```python
from build123d import *

# Parameters (mm, degrees)
CBORE_FOR_M2_SHCS1_AT_2_COUNT = 2
CBORE_FOR_M2_SHCS1_AT_2_PITCH = 6.363961031
CBORE_FOR_M2_SHCS1_AT_3_COUNT = 2
CBORE_FOR_M2_SHCS1_AT_3_PITCH = 9
CBORE_FOR_M2_SHCS1_AT_4_COUNT = 2
CBORE_FOR_M2_SHCS1_AT_4_PITCH = 6.363961031


with BuildPart() as part:
    # Sketch1 → Revolve1 (revolve)
    with BuildSketch(Plane.XY, mode=Mode.PRIVATE) as revolve1_sk:
        Polygon((0, 0), (8, 0), (8, 3.5), (2, 3.5), (2, 14.5), (0, 14.5), align=None)
    revolve(revolve1_sk.sketch.rotate(Axis((0, 14.5, 0), (0, -1, 0)), 180), axis=Axis((0, 14.5, 0), (0, -1, 0)))

    # Sketch4 → CBORE for M2 SHCS1 (revolve, cut)
    with BuildSketch(Plane(origin=(-4.5, 3.5, 0), x_dir=(0, 0, 1), z_dir=(1, 0, 0))):
        Polygon((0, 0), (0, 3.5), (1.2, 3.5), (1.2, 2), (2.2, 2), (2.2, 0.025), (2.225, 0), align=None)
    cbore_for_m2_shcs1 = revolve(axis=Axis((-4.5, 9.85, 0), (0, -1, 0)), mode=Mode.SUBTRACT)

    # CBORE for M2 SHCS1 at 2: CBORE for M2 SHCS1 ×2
    with Locations(*[Vector(0.7071067811865476, 0, -0.7071067811865476) * (i * CBORE_FOR_M2_SHCS1_AT_2_PITCH) for i in range(1, CBORE_FOR_M2_SHCS1_AT_2_COUNT)]):
        add(cbore_for_m2_shcs1, mode=Mode.SUBTRACT)

    # CBORE for M2 SHCS1 at 3: CBORE for M2 SHCS1 ×2
    with Locations(*[(i * CBORE_FOR_M2_SHCS1_AT_3_PITCH, 0, 0) for i in range(1, CBORE_FOR_M2_SHCS1_AT_3_COUNT)]):
        add(cbore_for_m2_shcs1, mode=Mode.SUBTRACT)

    # CBORE for M2 SHCS1 at 4: CBORE for M2 SHCS1 ×2
    with Locations(*[Vector(0.7071067811865476, 0, 0.7071067811865476) * (i * CBORE_FOR_M2_SHCS1_AT_4_PITCH) for i in range(1, CBORE_FOR_M2_SHCS1_AT_4_COUNT)]):
        add(cbore_for_m2_shcs1, mode=Mode.SUBTRACT)


solid = part.part
```
Could you check a few things on this model? Use its own coordinates, in mm. A direction names the side the tool comes from. Round coordinates to 2 decimals unless told otherwise and drop trailing zeros. Loops run counter-clockwise (first coordinate to the right, second up) from the corner with the lowest first, then second, coordinate; pieces in that order, holes last. Notation, with made-up numbers: (-14.75, 75.25) - (11.25, 75.25) arc R11 cw to (11.25, 92.25) - close; hole circle Ø1 at (-27.5, -23). An arc over 180 degrees is marked (long way). Use CSV: the item, a comma, the result in double quotes.
Item 1: If we section it at B-B on z = 4.5: List the corners of the cut face in (x, y) for me (3 decimals), then the cut area to 3 significant figures.
Here are the results:
outline,"(-6.614, 0) - (-1.2, 0) - (-1.2, 1.5) - (-2.2, 1.5) - (-2.2, 3.475) - (-2.225, 3.5) - (-6.614, 3.5) - close; (1.2, 0) - (6.614, 0) - (6.614, 3.5) - (2.225, 3.5) - (2.2, 3.475) - (2.2, 1.5) - (1.2, 1.5) - close"
area,"33.9 mm²"
Item 2: If we section it at A-A on z = 0: List the corners of the cut face in (x, y) for me (3 decimals), then the cut area to 3 significant figures.
Here are the results:
outline,"(-8, 0) - (-5.7, 0) - (-5.7, 1.5) - (-6.7, 1.5) - (-6.7, 3.475) - (-6.725, 3.5) - (-8, 3.5) - close; (-3.3, 0) - (3.3, 0) - (3.3, 1.5) - (2.3, 1.5) - (2.3, 3.475) - (2.275, 3.5) - (2, 3.5) - (2, 14.5) - (-2, 14.5) - (-2, 3.5) - (-2.275, 3.5) - (-2.3, 3.475) - (-2.3, 1.5) - (-3.3, 1.5) - close; (5.7, 0) - (8, 0) - (8, 3.5) - (6.725, 3.5) - (6.7, 3.475) - (6.7, 1.5) - (5.7, 1.5) - close"
area,"75.2 mm²"
Item 3: I need wall thicknesses on L1, parallel to Y at x = -1.5, z = 5; L2, parallel to Y at x = -2.25, z = 5.5; L3, parallel to X at y = 2.3, z = -4.5. Which ranges of each line are inside material? Lowest first, please. Write a range as [from, to].
Here are the results:
L1,"y = [0, 1.5]"
L2,"y = [0, 3.5]"
L3,"x = [-6.61, -2.2], [2.2, 6.61]"
Item 4: If we mould it in two halves opening along Z, with no side actions, what happens to faces 3 (the flat face through (0, 14.5, 0)), 4 (the cylindrical face through (-0.05, 0.76, 3.3)), 5 (the flat face through (-4.5, 1.5, -1.4)), 6 (the cylindrical face through (0, 9, 2))? For each: pulls with the +Z half, pulls with the -Z half, needs draft (parallel to the pull), parting line crosses it, or undercut.
Here are the results:
face 3,"needs draft"
face 4,"undercut"
face 5,"undercut"
face 6,"parting line crosses it"
Item 5: Will these pins go through, and if not, where does the flat tip stop? pin 1 (4 mm diameter, centred on x = 0, z = -4.5, fed in from -Y); pin 2 (5 mm diameter, centred on x = -6.5, y = 3.5, fed in from +Z); pin 3 (3.5 mm diameter, centred on x = -4, z = 0.5, fed in from +Y); pin 4 (3 mm diameter, centred on y = 3, z = 5.5, fed in from -X).
Here are the results:
pin 1,"stops at y = 0"
pin 2,"stops at z = 6.93"
pin 3,"stops at y = 3.5"
pin 4,"stops at x = -6.93"
Item 6: For faces 1 (the cylindrical face through (-0.05, 0.76, -5.7)), 2 (the cylindrical face through (2.32, 2.5, -0.29)), which set-ups out of +Z, -Z, +X, -X, +Y, -Y let a thin tool reach every point of the face, with its end or its side?
Here are the results:
face 1,"+Y, -Y"
face 2,"+Y"
Item 7: If we section it at C-C on x = -4.5: List the corners of the cut face in (y, z) for me (3 decimals), then the cut area to 3 significant figures.
Here are the results:
outline,"(0, -6.614) - (3.5, -6.614) - (3.5, -2.225) - (3.475, -2.2) - (1.5, -2.2) - (1.5, -1.2) - (0, -1.2) - close; (0, 1.2) - (1.5, 1.2) - (1.5, 2.2) - (3.475, 2.2) - (3.5, 2.225) - (3.5, 6.614) - (0, 6.614) - close"
area,"33.9 mm²"
Item 8: If we section it at D-D on y = 6.75: List the corners of the cut face in (x, z) for me, then the cut area to 3 significant figures.
Here are the results:
outline,"circle Ø4 at (0, 0)"
area,"12.6 mm²"
